Could you check a few things on this model? Use its own coordinates, in mm. A direction names the side the tool comes from. Coordinates: 2 decimals unless noted, no trailing zeros. Write each loop counter-clockwise with the first axis right and the second up, starting at its lowest first coordinate (ties: lowest second). Pieces come first, ordered by that corner, then holes.
Item 1: I want a section at A-A on x = 0. Please give me the cut outline in (y, z), then the cut area to 4 significant figures.
Item 2: I want a section at B-B on y = 7. Please give me the cut outline in (x, z), then the cut area to 3 significant figures.
Item 3: I want a section at D-D on z = 0. Please give me the cut outline in (x, y), then the cut area to 3 significant figures.
Item 4: For P1, Ø14, axis at x = 0.5, z = -1.5, coming from the -Y side; P2, Ø10, axis at y = 11.5, z = 2, coming from the +X side; P3, Ø8.5, axis at x = -27, z = -12, coming from the +Y side; P4, Ø4.5, axis at y = 10.5, z = -3.5, coming from the -X side, each with a flat end and sliding along its axis, tell me the tip position at first contact or that it passes through.
Item 5: If I drill on probe 1 along X at (y, z) = (29, -10); probe 2 along Z at (x, y) = (10, 30); probe 3 along Z at (x, y) = (-10.15, 30.8), over which ranges is the centre line in solid material (lowest first)?
Item 6: Thinking about a two-plate mould opening in X: for faces 1 (the cylindrical face through (9.942, 29.979, -8.564)), 2 (the flat face through (-31, 2, -23)), 3 (the cylindrical face through (-20.9, 3.86, -10.88)), which applies, +X half, -X half, draft (parallel to the pull), parting line (faces both ways), or undercut?
Item 7: I want a section at C-C on z = -11. Please give me the cut outline in (x, y).
Item 8: Which directions (+Z, -Z, +X, -X, +Y, -Y) give clear straight access to the entire face, cutting with the end or side of a thin tool? Please do faces 4 (the cylindrical face through (-17.86, 0.9, -9.75)), 5 (the flat face through (-20, 22, -10)), 6 (the flat face through (18, 27.5, -21)), 7 (the cylindrical face through (-28.236, 1.479, -12.516)), 8 (the flat face through (17, 27.5, 10)).
from build123d import *

# Parameters (mm, degrees)
PAD_DEPTH            = 21
PAD_DEPTH_BACK       = 23
POCKET_DEPTH         = 27.5
POCKET001_DEPTH      = 31.501
POCKET002_DEPTH      = 33.78525
POCKET002_DEPTH_BACK = -33.78525
SKETCH004_R          = 1.6
SKETCH004_R_2        = 8.1
POCKET003_DEPTH      = 31.501
CHAMFER_SIZE         = 1.5
FILLET_R             = 3


with BuildPart() as part:
    # Sketch → Pad (new body, two sides)
    with BuildSketch(Plane.XY) as pad_sk:
        with BuildLine():
            Line((-33.78425, 0), (-17, 0))
            Line((-17, 0), (-17, 25.5))
            ThreePointArc((-14, 28.5), (-16.12132, 27.62132), (-17, 25.5))
            Line((-14, 28.5), (14, 28.5))
            ThreePointArc((17, 25.5), (16.12132, 27.62132), (14, 28.5))
            Line((17, 25.5), (17, 0))
            Line((17, 0), (33.78425, 0))
            Line((33.78425, 0), (33.78425, 3))
            Line((23, 3), (33.78425, 3))
            ThreePointArc((20, 6), (20.87868, 3.87868), (23, 3))
            Line((20, 31.5), (20, 6))
            Line((-20, 31.5), (20, 31.5))
            Line((-20, 31.5), (-20, 6))
            ThreePointArc((-23, 3), (-20.87868, 3.87868), (-20, 6))
            Line((-33.78425, 3), (-23, 3))
            Line((-33.78425, 0), (-33.78425, 3))
        make_face()
    extrude(amount=PAD_DEPTH)
    extrude(pad_sk.sketch, amount=-PAD_DEPTH_BACK)

    # Sketch001 → Pocket (cut)
    with BuildSketch(Plane.XZ):
        with BuildLine():
            ThreePointArc((26.084271, -17.715729), (28.284271, -19.915729), (30.484271, -17.715729))
            Line((30.484271, -17.715729), (30.484271, -14.715729))
            ThreePointArc((30.484271, -14.715729), (28.284271, -12.515729), (26.084271, -14.715729))
            Line((26.084271, -17.715729), (26.084271, -14.715729))
        make_face()
        with BuildLine():
            ThreePointArc((-26.084271, -14.715729), (-28.284271, -12.515729), (-30.484271, -14.715729))
            Line((-30.484271, -14.715729), (-30.484271, -17.715729))
            ThreePointArc((-30.484271, -17.715729), (-28.284271, -19.915729), (-26.084271, -17.715729))
            Line((-26.084271, -14.715729), (-26.084271, -17.715729))
        make_face()
        with BuildLine():
            Line((-35.5, -45), (35.5, -45))
            ThreePointArc((35.5, -45), (25.102291, -19.897709), (0, -9.5))
            ThreePointArc((0, -9.5), (-25.102291, -19.897709), (-35.5, -45))
        make_face()
    extrude(amount=-POCKET_DEPTH, mode=Mode.SUBTRACT)

    # Sketch002 → Pocket001 (cut, through all)
    with BuildSketch(Plane.XZ):
        with BuildLine():
            ThreePointArc((21, 0), (0, 21), (-21, 0))
            Line((-21, -4), (-21, 0))
            Line((-38, -4), (-21, -4))
            Line((-38, 34), (-38, -4))
            Line((38, 34), (-38, 34))
            Line((38, -4), (38, 34))
            Line((21, -4), (38, -4))
            Line((21, 0), (21, -4))
        make_face()
    extrude(amount=-POCKET001_DEPTH, mode=Mode.SUBTRACT)

    # Sketch005 → Pocket002 (cut, two sides)
    with BuildSketch(Plane.YZ) as pocket002_sk:
        with BuildLine():
            Line((0, -4), (15.5, -4))
            ThreePointArc((15.5, -4), (23.985281, -0.485281), (27.5, 8))
            Line((27.5, 8), (27.5, 26))
            Line((27.5, 26), (0, 26))
            Line((0, 26), (0, -4))
        make_face()
    extrude(amount=-POCKET002_DEPTH, mode=Mode.SUBTRACT)
    extrude(pocket002_sk.sketch, amount=-POCKET002_DEPTH_BACK, mode=Mode.SUBTRACT)

    # Sketch004 → Pocket003 (cut, through all)
    with BuildSketch(Plane.XZ):
        with Locations((-10.15, 10.15)):
            Circle(SKETCH004_R)
        with Locations((10.15, 10.15)):
            Circle(SKETCH004_R)
        with Locations((10.15, -10.15)):
            Circle(SKETCH004_R)
        with Locations((-10.15, -10.15)):
            Circle(SKETCH004_R)
        Circle(SKETCH004_R_2)
    extrude(amount=-POCKET003_DEPTH, mode=Mode.SUBTRACT)

    # Chamfer
    chamfer_edges = [part.edges().sort_by_distance(p)[0] for p in [
        (-8.1, 31.5, 0),
    ]]
    chamfer(chamfer_edges, length=CHAMFER_SIZE)

    # Fillet
    fillet_edges = [part.edges().sort_by_distance(p)[0] for p in [
        (33.78425, 1.5, -4),
        (-33.78425, 1.5, -4),
        (-20, 29.5, -23),
        (20, 29.5, -23),
        (-17, 0, -8.917558),
        (17, 0, -8.917558),
        (-18.152606, 27.5, -14.492085),
        (18.152606, 27.5, -14.492085),
    ]]
    fillet(fillet_edges, radius=FILLET_R)


solid = part.part
Response values:
1. outline: (28.5, -23) - (31.5, -23) - (31.5, -9.6) - (30, -8.1) - (28.5, -8.1) - close; (28.5, 8.1) - (30, 8.1) - (31.5, 9.6) - (31.5, 21) - (28.5, 21) - close
1. area: 81.15 mm2
2. outline: (-20, -15.67) arc R35.5 cw to (-17, -13.84) - (-17, -4) - (-20, -4) - close; (17, -13.84) arc R35.5 cw to (20, -15.67) - (20, -4) - (17, -4) - close
2. area: 64.3 mm2
3. outline: (-20, 24.44) - (-17, 24.44) - (-17, 25.5) arc R3 cw to (-14, 28.5) - (-8.1, 28.5) - (-8.1, 30) - (-9.6, 31.5) - (-20, 31.5) - close; (8.1, 28.5) - (14, 28.5) arc R3 cw to (17, 25.5) - (17, 24.44) - (20, 24.44) - (20, 31.5) - (9.6, 31.5) - (8.1, 30) - close
3. area: 97.3 mm2
4. P1: stops at y = 28.5
4. P2: passes through
4. P3: stops at y = 3.01
4. P4: stops at x = -20
5. probe 1: x = -20 to -11.74, -8.56 to 8.56, 11.74 to 20
5. probe 2: z = -23 to -11.74, -8.56 to 8.56, 11.74 to 18.47
5. probe 3: z = -23 to -11.75, -8.55 to 8.55, 11.75 to 18.38
6. face 1: undercut
6. face 2: draft
6. face 3: -X half
7. outline: (-33.78, 0) - (-20, 0) arc R3 ccw to (-17, 3) - (-17, 25.5) arc R3 cw to (-14, 28.5) - (-11.51, 28.5) - (-11.51, 31.5) - (-20, 31.5) - (-20, 6) arc R3 cw to (-23, 3) - (-33.78, 3) - close; (-8.79, 28.5) - (8.79, 28.5) - (8.79, 31.5) - (-8.79, 31.5) - close; (11.51, 28.5) - (14, 28.5) arc R3 cw to (17, 25.5) - (17, 3) arc R3 ccw to (20, 0) - (33.78, 0) - (33.78, 3) - (23, 3) arc R3 cw to (20, 6) - (20, 31.5) - (11.51, 31.5) - close
8. face 4: +Z, -Z, -Y
8. face 5: +Z, -Z, -X, +Y
8. face 6: -Z, -Y
8. face 7: +Y, -Y
8. face 8: +Z, +X, -X, -Y
